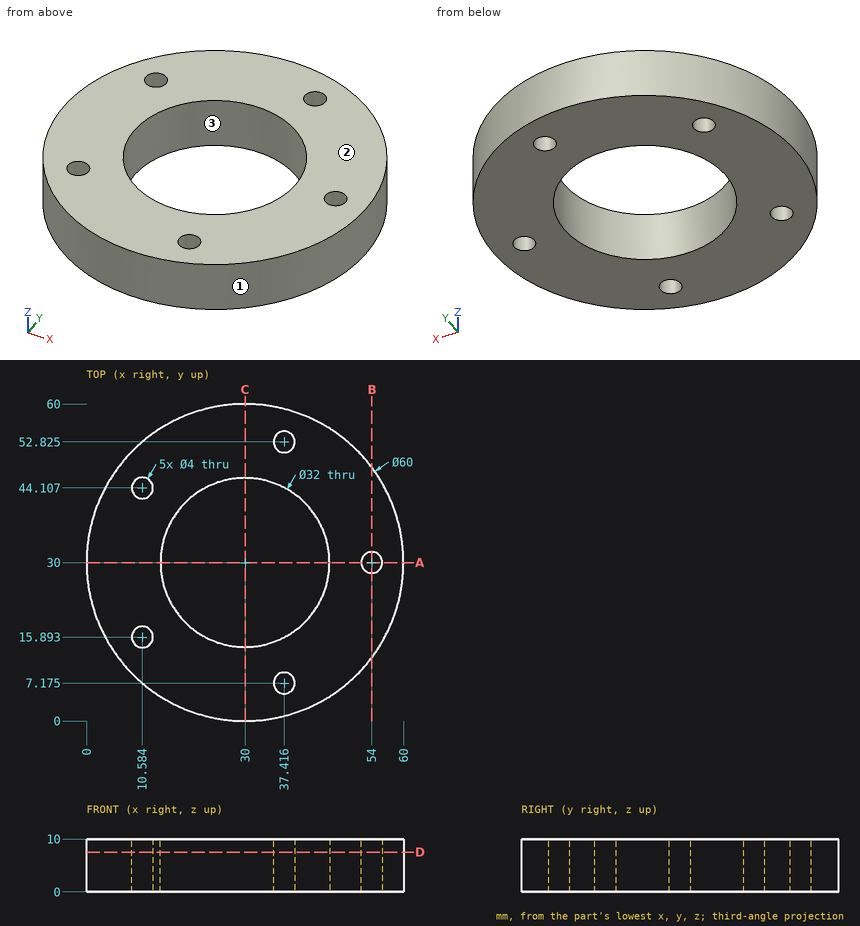
The figure shows three views and two pictorial views of one solid part (mm, origin at its lowest corner). Answer the questions. Round coordinates to 2 decimals unless told otherwise and drop trailing zeros. Order: outer loops, then holes, each group sorted by start corner. A loop starts at its lowest first (then second) coordinate and runs counter-clockwise, first axis right, second up.
Q1. A cutting plane is placed at C-C, the plane x = 30. Determine the outline of the cut face in (y, z).
Solution:
outline: (0, 0) - (14, 0) - (14, 10) - (0, 10) - close; (46, 0) - (60, 0) - (60, 10) - (46, 10) - close
Q2. The mould has two halves that part along X. Classify the marked faces 1, 2 and 3: pulls with the +X half, pulls with the -X half, needs draft (parallel to the pull), parting line crosses it, or undercut.
Solution:
face 1: parting line crosses it
face 2: needs draft
face 3: undercut
Q3. A cutting plane is placed at D-D, the plane z = 7.5. Determine the outline of the cut face in (x, y) (1 decimal), then the cut area to 3 significant figures.
Solution:
outline: circle Ø60 at (30, 30); hole circle Ø4 at (10.6, 15.9); hole circle Ø4 at (10.6, 44.1); hole circle Ø32 at (30, 30); hole circle Ø4 at (37.4, 7.2); hole circle Ø4 at (37.4, 52.8); hole circle Ø4 at (54, 30)
area: 1,960 mm2
Q4. Given pin 1 Ø3 at (y, z) = (52, 7) entering from +X; pin 2 Ø3 at (x, y) = (54, 30) entering from -Z; pin 3 Ø3 at (y, z) = (36, 9) entering from -X, each flat-ended and moving along its own axis, determine where each tip first touches the part or whether it passes through.
Solution:
pin 1: stops at x = 51.9
pin 2: passes through
pin 3: stops at x = 0.34
Q5. A cutting plane is placed at A-A, the plane y = 30. Determine the outline of the cut face in (x, z), then the cut area to 3 significant figures.
Solution:
outline: (0, 0) - (14, 0) - (14, 10) - (0, 10) - close; (46, 0) - (52, 0) - (52, 10) - (46, 10) - close; (56, 0) - (60, 0) - (60, 10) - (56, 10) - close
area: 240 mm2
Q6. A cutting plane is placed at B-B, the plane x = 54. Determine the outline of the cut face in (y, z).
Solution:
outline: (12, 0) - (28, 0) - (28, 10) - (12, 10) - close; (32, 0) - (48, 0) - (48, 10) - (32, 10) - close
Q7. Find the intervals of material crossed by line 1 along Y through (x, z) = (10.5, 4.75) (1 decimal); line 2 along Y through (x, z) = (30.5, 5.75) (1 decimal); line 3 along Y through (x, z) = (11.5, 0.75) (1 decimal), in increasing order.
Solution:
line 1: y = 7.2 to 13.9, 17.9 to 42.1, 46.1 to 52.8
line 2: y = 0 to 14, 46 to 60
line 3: y = 6.4 to 14.1, 17.7 to 42.3, 45.9 to 53.6
